Autodesk Inventor part; units mm, degrees
ref_plane "YZ Plane" through (0, 0, 0) normal (1, 0, 0) x (0, 1, 0)
ref_plane "XZ Plane" through (0, 0, 0) normal (0, 1, 0) x (-1, 0, 0)
ref_plane "XY Plane" through (0, 0, 0) normal (0, 0, 1) x (1, 0, 0)
sketch "Sketch1" plane through (0, 0, 0) normal (0, 1, 0) x (-1, 0, 0)
  line L0 (0, 0) -> (-22.86, 0)
  line L1 (-22.86, 0) -> (-22.86, -22.86)
  line L2 (-22.86, -22.86) -> (0, -22.86)
  line L3 (0, -22.86) -> (0, 0)
  line L4 (-22.86, -22.86) -> (-19.304, -22.86)
  line L5 (-19.304, -22.86) -> (-19.304, -19.304) construction
  line L6 (-19.304, -19.304) -> (-22.86, -19.304) construction
  line L7 (-22.86, -19.304) -> (-22.86, -22.86)
  line L8 (0, -22.86) -> (-3.556, -22.86)
  line L9 (-3.556, -22.86) -> (-3.556, -19.304) construction
  line L10 (-3.556, -19.304) -> (0, -19.304) construction
  line L11 (0, -19.304) -> (0, -22.86)
  line L12 (0, 0) -> (-3.556, 0)
  line L13 (-3.556, 0) -> (-3.556, -3.556) construction
  line L14 (-3.556, -3.556) -> (0, -3.556) construction
  line L15 (0, -3.556) -> (0, 0)
  line L16 (-22.86, 0) -> (-19.304, 0)
  line L17 (-19.304, 0) -> (-19.304, -3.556) construction
  line L18 (-19.304, -3.556) -> (-22.86, -3.556) construction
  line L19 (-22.86, -3.556) -> (-22.86, 0)
  circle A0 centre (-3.556, -19.304) radius 2.032
  circle A1 centre (-19.304, -19.304) radius 2.032
  circle A2 centre (-19.304, -3.556) radius 2.032
  circle A3 centre (-3.556, -3.556) radius 2.032
  line L20 (3.57, -26.43) -> (-26.43, -26.43)
  line L21 (-26.43, -26.43) -> (-26.43, 3.57)
  line L22 (-26.43, 3.57) -> (3.57, 3.57)
  line L23 (3.57, 3.57) -> (3.57, -26.43)
  line L24 (0, 0) -> (-6.5, 0)
  line L25 (-6.5, 0) -> (-6.5, -6.5)
  line L26 (-6.5, -6.5) -> (0, -6.5)
  line L27 (0, -6.5) -> (0, 0)
  line L28 (0, -22.86) -> (-6.5, -22.86)
  line L29 (-6.5, -22.86) -> (-6.5, -16.36)
  line L30 (-6.5, -16.36) -> (0, -16.36)
  line L31 (0, -16.36) -> (0, -22.86)
  line L32 (-22.86, -22.86) -> (-16.36, -22.86)
  line L33 (-16.36, -22.86) -> (-16.36, -16.36)
  line L34 (-16.36, -16.36) -> (-22.86, -16.36)
  line L35 (-22.86, -16.36) -> (-22.86, -22.86)
  line L36 (-22.86, 0) -> (-16.36, 0)
  line L37 (-16.36, 0) -> (-16.36, -6.5)
  line L38 (-16.36, -6.5) -> (-22.86, -6.5)
  line L39 (-22.86, -6.5) -> (-22.86, 0)
  line L40 (-26.43, 3.57) -> (-68.4276, 3.57)
  line L41 (-68.4276, 3.57) -> (-68.4276, -26.43)
  line L42 (-68.4276, -26.43) -> (-26.43, -26.43)
  line L43 (-26.43, -26.43) -> (-26.43, 3.57)
  circle A4 centre (-11.43, -11.43) radius 5
  point P0 (0, -16.36)
  point P1 (0, -6.5)
  dimension "d2" = 22.86
  dimension "d3" = 22.86
  dimension "d4" = 3.556
  dimension "d5" = 3.556
  dimension "d6" = 3.556
  dimension "d7" = 3.556
  dimension "d8" = 3.556
  dimension "d9" = 3.556
  dimension "d10" = 3.556
  dimension "d11" = 3.556
  dimension "d12" = 4.064
  dimension "d13" = 4.064
  dimension "d14" = 4.064
  dimension "d15" = 4.064
  dimension "d16" = 30
  dimension "d17" = 30
  dimension "d18" = 3.57
  dimension "d19" = 3.57
  dimension "d20" = 6.5
  dimension "d21" = 6.5
  dimension "d22" = 6.5
  dimension "d23" = 6.5
  dimension "d24" = 6.5
  dimension "d25" = 6.5
  dimension "d26" = 6.5
  dimension "d31" = 10
  dimension "d32" = 15
  dimension "d33" = 15
  dimension "d34" = 56.9976
extrude "Extrusion1" add sketch "Sketch1" along normal blind 7 contours L3 L26 L25 L0 | L37 L38 L1 L0 | L3 L2 L29 L30 | L34 L33 L2 L1 | L20 L21 L22 L23 | L42 L41 L40 L21
fillet "Fillet1" radius 2 4 edges at (6.5, 3.5, -16.36) (16.36, 3.5, -16.36) (16.36, 3.5, -6.5) (6.5, 3.5, -6.5)
sketch "Sketch4" plane through (68.4276, 0, 3.57) normal (1, 0, 0) x (0, 0, -1)
  line L0 (-15, 13.5061) -> (45, 13.5061)
  line L1 (45, 13.5061) -> (45, -6.4939)
  line L2 (45, -6.4939) -> (-15, -6.4939)
  line L3 (-15, -6.4939) -> (-15, 13.5061)
  line L4 (-15, 13.5061) -> (45, -6.4939) construction
  line L5 (45, 13.5061) -> (-15, -6.4939) construction
  line L6 (30, 0) -> (30, 7)
  line L7 (15, 3.5061) -> (39, 3.5061)
  circle A0 centre (39, 3.5061) radius 2.8838
  circle A1 centre (-9, 3.5061) radius 2.421
  line L8 (-15, 0) -> (45, 0)
  line L9 (45, 0) -> (45, 13.5061)
  line L10 (45, 13.5061) -> (-15, 13.5061)
  line L11 (-15, 13.5061) -> (-15, 0)
  point P0 (3.57, 0)
  dimension "d46" = 60
  dimension "d47" = 20
  dimension "d48" = 15
  dimension "d49" = 10
  dimension "d56" = 24
  dimension "d57" = 24
extrude "Extrusion4" add sketch "Sketch4" against normal blind 5 contours L0 L1 L8 L3
properties part number "as5600mount"
The model under review builds one solid part; all positions refer to its coordinate system, in mm. A direction names the side the tool comes from. Give positions to 0.01 mm unless a question says otherwise; leave off trailing zeros. Order: outer loops, then holes, each group sorted by start corner. A loop starts at its lowest first (then second) coordinate and runs counter-clockwise, first axis right, second up. Notation, with made-up numbers: M 18.5,-34 L 66.5,-34 A31 cw 66.5,-3 Z; hole C 43.25,73.25 d8. An arc over 180 degrees is marked long. Use one line per item in the form item = value. Start each with the question number.
Item 1: We need section D-D on y = 8.75. Give the boundary of the cut face in (x, z).
Item 2: We need section A-A on z = 12.57. Give the boundary of the cut face in (x, y), plus the area to 3 significant figures.
Item 3: We need section C-C on z = 1. Give the boundary of the cut face in (x, y), plus the area to 3 significant figures.
Item 4: We need section B-B on x = 10.5. Give the boundary of the cut face in (y, z), plus the area to 3 significant figures.
Item 5: The part is to be moulded in two halves that separate along Z. For faces 3 (the flat face through (30, 3, 3.57)), 4 (the flat face through (66, 13.506, -11)), 5 (the flat face through (0, 3, -11)), say which applies: pulls with the +Z half, pulls with the -Z half, needs draft (parallel to the pull), parting line crosses it, or undercut.
Item 6: For faces 1 (the flat face through (41, 0, -11)), 2 (the cylindrical face through (16.93, 3.55, -16.96)), list the 3-axis set-ups (+Z, -Z, +X, -X, +Y, -Y) from which the entire face can be reached by the end or side of a thin tool; tool diameter is ignored.
Item 7: To check wall thickness, follow line 1 along X through (y, z) = (3.75, -16); line 2 along Z through (x, y) = (14, 6.75); line 3 along Y through (x, z) = (30, -16). State the ranges of each line that lie inside material, in increasing order. Write a range as from..to.
Item 8: Insertion check: pin 1 Ø3.5 at (x, y) = (22.5, 5) entering from -Z; pin 2 Ø24 at (x, z) = (21.5, -5) entering from +Y; pin 3 Ø3 at (y, z) = (10.5, -10) entering from -X. Each pin has a flat end and moves straight along its axis. Give the tip position at first contact, or say it passes through.
Completed:
q1.outline = M 63.43,-41.43 L 68.43,-41.43 L 68.43,18.57 L 63.43,18.57 Z
q2.outline = M 63.43,0 L 68.43,0 L 68.43,1.09 L 63.43,1.09 Z; M 63.43,5.93 L 68.43,5.93 L 68.43,13.51 L 63.43,13.51 Z
q2.area = 43.3 mm²
q3.outline = M -3.57,0 L 68.43,0 L 68.43,13.51 L 63.43,13.51 L 63.43,7 L -3.57,7 Z
q3.area = 537 mm²
q4.outline = M 0,-26.43 L 7,-26.43 L 7,-22.86 L 0,-22.86 Z; M 0,0 L 7,0 L 7,3.57 L 0,3.57 Z
q4.area = 50.0 mm²
q5.face_3 = pulls with the +Z half
q5.face_4 = needs draft
q5.face_5 = undercut
q6.face_1 = +Z, -Z, +X, -X, -Y
q6.face_2 = +Y, -Y
q7.line_1 = -3.57..0, 22.86..68.43
q7.line_2 = -26.43..-22.86, 0..3.57
q7.line_3 = 0..7
q8.pin_1 = -26.43
q8.pin_2 = 7
q8.pin_3 = 63.43
